Part model, mm, in its own coordinate system. Face numbers are marked on the shaded views. A direction names the side the tool comes from. Coordinates: 2 decimals unless noted, no trailing zeros. Order: outer loops, then holes, each group sorted by start corner. A loop starts at its lowest first (then second) coordinate and runs counter-clockwise, first axis right, second up.
1) Cut at A-A (x = -10). List the corners of the cut face in (y, z), and give its area (3 significant figures).
2) Cut at B-B (y = 69). List the corners of the cut face in (x, z), and give its area (3 significant figures).
3) Pin check, flat tips, straight feed: pin 1 Ø1.5 at (x, z) = (-19, 4.5) entering from -Y; pin 2 Ø8 at (x, y) = (12.5, 48.5) entering from +Z; pin 3 Ø4 at (y, z) = (45, 9) entering from +X. Stop position of each tip, or through.
4) Tool access for the marked faces 1, 2, 3, 4 and 5: list every direction of +Z, -Z, +X, -X, +Y, -Y with a clear straight run to the whole face (end or side of a thin tool).
5) Wall check: L1, parallel to X at y = 37, z = 5.5; L2, parallel to Y at x = 18, z = 3.5; L3, parallel to Z at x = 25.5, y = 56.5. Give the ranges that are in metal, low to high.
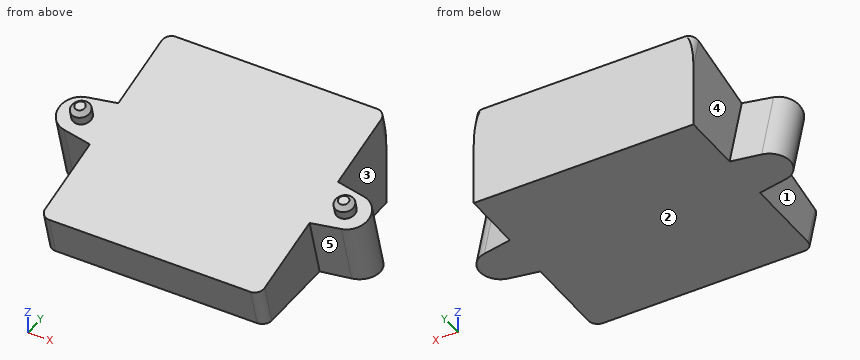
```python
from build123d import *

# Parameters (mm, degrees)
F1_DEPTH = 34.25
F2_R     = 2.1
F3_DEPTH = 30
F5_DEPTH = 3
F6_SIZE  = 1


with BuildPart() as f1:
    # F0 (on Right) → F1 (new body, symmetric)
    with BuildSketch(Plane.YZ):
        Polygon((81.137769, 21.7408), (0, 0), (81.137769, 0), align=None)
    extrude(amount=F1_DEPTH, both=True)


with BuildPart() as f3:
    # F2 (on face) → F3 (new body)
    with BuildSketch(Plane(origin=(0, 0, 0), x_dir=(1, 0, 0), z_dir=(0, -0.258819, 0.965926))):
        with BuildLine():
            Line((-22.25, 35), (0, 35))
            Line((0, 35), (0, 84))
            Line((0, 84), (-22.25, 84))
            ThreePointArc((-22.25, 84), (-23.664214, 83.414214), (-24.25, 82))
            Line((-24.25, 82), (-24.25, 65.318283))
            Line((-24.25, 65.318283), (-30.615681, 64.16811))
            ThreePointArc((-30.615681, 64.16811), (-34.25, 59.818283), (-30.615681, 55.468456))
            Line((-30.615681, 55.468456), (-24.25, 54.318283))
            Line((-24.25, 54.318283), (-24.25, 37))
            ThreePointArc((-24.25, 37), (-23.664214, 35.585786), (-22.25, 35))
        make_face()
        with Locations((-29.1, 59.818283)):
            Circle(F2_R, mode=Mode.SUBTRACT)
        with BuildLine():
            Line((0, 84), (0, 35))
            Line((0, 35), (22.25, 35))
            ThreePointArc((22.25, 35), (23.664214, 35.585786), (24.25, 37))
            Line((24.25, 37), (24.25, 54.318283))
            Line((24.25, 54.318283), (30.615681, 55.468456))
            ThreePointArc((30.615681, 55.468456), (34.25, 59.818283), (30.615681, 64.16811))
            Line((30.615681, 64.16811), (24.25, 65.318283))
            Line((24.25, 65.318283), (24.25, 82))
            ThreePointArc((24.25, 82), (23.664214, 83.414214), (22.25, 84))
            Line((22.25, 84), (0, 84))
        make_face()
        with Locations((29.1, 59.818283)):
            Circle(F2_R, mode=Mode.SUBTRACT)
        with Locations((29.1, 59.818283)):
            Circle(F2_R)
        with Locations((-29.1, 59.818283)):
            Circle(F2_R)
    extrude(amount=-F3_DEPTH)

    # F4: intersect F1
    add(f1.part, mode=Mode.INTERSECT)

    # F2 (on face) → F5 (join)
    with BuildSketch(Plane(origin=(0, 0, 0), x_dir=(1, 0, 0), z_dir=(0, -0.258819, 0.965926))):
        with Locations((29.1, 59.818283)):
            Circle(F2_R)
        with Locations((-29.1, 59.818283)):
            Circle(F2_R)
    extrude(amount=F5_DEPTH)

    # F6
    f6_edges = [f3.edges().sort_by_distance(p)[0] for p in [
        (27, 57.003567, 18.379888),
        (-31.2, 57.003567, 18.379888),
    ]]
    chamfer(f6_edges, length=F6_SIZE)


solid = f3.part
```
Geometry check:
1. outline: (33.81, 9.06) - (36.23, 0) - (81.14, 0) - (81.14, 21.74) - close
1. area: 718 mm2
2. outline: (-24.25, 0) - (24.25, 0) - (24.25, 18.49) - (-24.25, 18.49) - close
2. area: 897 mm2
3. pin 1: stops at y = 34.83
3. pin 2: stops at z = 14.07
3. pin 3: stops at x = 24.25
4. face 1: -Z, -X, -Y
4. face 2: -Z, +X, -X, +Y, -Y
4. face 3: +Z, +X, +Y
4. face 4: +Z, -X, +Y
4. face 5: -Z, +X, -Y
5. L1: x = -24.25 to 24.25
5. L2: y = 35.3 to 81.14
5. L3: z = 0 to 15.14
